```python
from build123d import *

# Parameters (mm, degrees)
BOSS_EXTRUDE1_DEPTH            = 6
CBORE_FOR_M6_SHCS1_D           = 7
CBORE_FOR_M6_SHCS1_CBORE_D     = 10.5
CBORE_FOR_M6_SHCS1_CBORE_DEPTH = 5
FILLET1_R                      = 1


with BuildPart() as part:
    # Sketch1 → Boss-Extrude1 (new, symmetric)
    with BuildSketch(Plane.XY):
        Polygon((-15, 13), (-15, 3), (-4, 3), (-4, 0), (4, 0), (4, 3), (15, 3), (15, 13), align=None)
    extrude(amount=BOSS_EXTRUDE1_DEPTH, both=True)

    # CBORE for M6 SHCS1 (through all)
    with Locations(Plane(origin=(0, 13, 0), x_dir=(1, 0, 0), z_dir=(0, 1, 0))):
        with Locations((0, 0)):
            CounterBoreHole(CBORE_FOR_M6_SHCS1_D / 2, CBORE_FOR_M6_SHCS1_CBORE_D / 2, CBORE_FOR_M6_SHCS1_CBORE_DEPTH)

    # Fillet1
    # the kernel refuses this fillet: 1 mm, written as the material it takes off along each edge
    with BuildSketch(Plane(origin=(-3, 1, 5), x_dir=(-1, 0, 0), z_dir=(0, 0, 1))) as fillet1_piece_1_section:
        Polygon((0, 0), (FILLET1_R, 0), (FILLET1_R, FILLET1_R), (0, FILLET1_R), align=None)
    fillet1_piece_1 = extrude(amount=FILLET1_R, mode=Mode.PRIVATE)
    fillet1_piece_1 = fillet1_piece_1 - Plane(origin=(-3, 1, 5), x_dir=(0.7071067811865475, 0.7071067811865475, 0), z_dir=(0, 0, 1)) * Sphere(FILLET1_R, mode=Mode.PRIVATE)
    add(fillet1_piece_1, mode=Mode.SUBTRACT)
    with BuildSketch(Plane(origin=(3, 1, -5), x_dir=(0, -1, 0), z_dir=(0, 0, -1))) as fillet1_piece_2_section:
        Polygon((0, 0), (FILLET1_R, 0), (FILLET1_R, -FILLET1_R), (0, -FILLET1_R), align=None)
    fillet1_piece_2 = extrude(amount=FILLET1_R, mode=Mode.PRIVATE)
    fillet1_piece_2 = fillet1_piece_2 - Plane(origin=(3, 1, -5), x_dir=(-0.7071067811865475, 0.7071067811865475, 0), z_dir=(0, 0, -1)) * Sphere(FILLET1_R, mode=Mode.PRIVATE)
    add(fillet1_piece_2, mode=Mode.SUBTRACT)
    with BuildSketch(Plane(origin=(3, 1, 5), x_dir=(0, -1, 0), z_dir=(0, 0, 1))) as fillet1_piece_3_section:
        Polygon((0, 0), (FILLET1_R, 0), (FILLET1_R, FILLET1_R), (0, FILLET1_R), align=None)
    fillet1_piece_3 = extrude(amount=FILLET1_R, mode=Mode.PRIVATE)
    fillet1_piece_3 = fillet1_piece_3 - Plane(origin=(3, 1, 5), x_dir=(-0.7071067811865475, 0.7071067811865475, 0), z_dir=(0, 0, 1)) * Sphere(FILLET1_R, mode=Mode.PRIVATE)
    add(fillet1_piece_3, mode=Mode.SUBTRACT)
    with BuildSketch(Plane(origin=(-3, 1, -5), x_dir=(-1, 0, 0), z_dir=(0, 0, -1))) as fillet1_piece_4_section:
        Polygon((0, 0), (FILLET1_R, 0), (FILLET1_R, -FILLET1_R), (0, -FILLET1_R), align=None)
    fillet1_piece_4 = extrude(amount=FILLET1_R, mode=Mode.PRIVATE)
    fillet1_piece_4 = fillet1_piece_4 - Plane(origin=(-3, 1, -5), x_dir=(0.7071067811865475, 0.7071067811865475, 0), z_dir=(0, 0, -1)) * Sphere(FILLET1_R, mode=Mode.PRIVATE)
    add(fillet1_piece_4, mode=Mode.SUBTRACT)
    with BuildSketch(Plane(origin=(-15, 15.5, -6), x_dir=(0, 0, 1), z_dir=(0, -1, 0)), Plane(origin=(15, 0.5, 6), x_dir=(-1, 0, 0), z_dir=(0, 1, 0))) as fillet1_piece_5:
        with BuildLine():
            CenterArc((FILLET1_R, -FILLET1_R), FILLET1_R, 90, 90)
            Line((0, -FILLET1_R), (0, 0))
            Line((0, 0), (FILLET1_R, 0))
        make_face()
    extrude(amount=15, mode=Mode.SUBTRACT)
    with BuildSketch(Plane(origin=(-4, 3, 6), x_dir=(1, 0, 0), z_dir=(0, -1, 0)), Plane(origin=(4, 1, 6), x_dir=(-1, 0, 0), z_dir=(0, 1, 0))) as fillet1_piece_6:
        with BuildLine():
            CenterArc((FILLET1_R, -FILLET1_R), FILLET1_R, 90, 90)
            Line((0, -FILLET1_R), (0, 0))
            Line((0, 0), (FILLET1_R, 0))
        make_face()
    extrude(amount=2, mode=Mode.SUBTRACT)
    with BuildSketch(Plane(origin=(4, 0, -5), x_dir=(-1, 0, 0), z_dir=(0, 0, 1)), Plane(origin=(-4, 0, -5), x_dir=(0, 1, 0), z_dir=(0, 0, 1))) as fillet1_piece_7:
        with BuildLine():
            CenterArc((FILLET1_R, -FILLET1_R), FILLET1_R, 90, 90)
            Line((0, -FILLET1_R), (0, 0))
            Line((0, 0), (FILLET1_R, 0))
        make_face()
    extrude(amount=10, mode=Mode.SUBTRACT)
    with BuildSketch(Plane(origin=(-3, 0, 6), x_dir=(0, 1, 0), z_dir=(1, 0, 0))) as fillet1_piece_8:
        with BuildLine():
            CenterArc((FILLET1_R, -FILLET1_R), FILLET1_R, 90, 90)
            Line((0, -FILLET1_R), (0, 0))
            Line((0, 0), (FILLET1_R, 0))
        make_face()
    extrude(amount=6, mode=Mode.SUBTRACT)
    with BuildSketch(Plane(origin=(-15, 15.5, 6), x_dir=(0, 0, -1), z_dir=(0, -1, 0)), Plane(origin=(15, 0.5, -6), x_dir=(-1, 0, 0), z_dir=(0, 1, 0))) as fillet1_piece_9:
        with BuildLine():
            CenterArc((FILLET1_R, FILLET1_R), FILLET1_R, 180, 90)
            Line((0, FILLET1_R), (0, 0))
            Line((0, 0), (FILLET1_R, 0))
        make_face()
    extrude(amount=15, mode=Mode.SUBTRACT)
    with BuildSketch(Plane(origin=(4, 1, -6), x_dir=(-1, 0, 0), z_dir=(0, 1, 0)), Plane(origin=(-4, 3, -6), x_dir=(1, 0, 0), z_dir=(0, -1, 0))) as fillet1_piece_10:
        with BuildLine():
            CenterArc((FILLET1_R, FILLET1_R), FILLET1_R, 180, 90)
            Line((0, FILLET1_R), (0, 0))
            Line((0, 0), (FILLET1_R, 0))
        make_face()
    extrude(amount=2, mode=Mode.SUBTRACT)
    with BuildSketch(Plane(origin=(-3, 0, -6), x_dir=(0, 1, 0), z_dir=(1, 0, 0))) as fillet1_piece_11:
        with BuildLine():
            CenterArc((FILLET1_R, FILLET1_R), FILLET1_R, 180, 90)
            Line((0, FILLET1_R), (0, 0))
            Line((0, 0), (FILLET1_R, 0))
        make_face()
    extrude(amount=6, mode=Mode.SUBTRACT)


solid = part.part
```
Input: part model. Units: mm. Frame: model coordinates. A direction names the side the tool comes from. Round coordinates to 2 decimals unless told otherwise and drop trailing zeros. Loops run counter-clockwise (first coordinate to the right, second up) from the corner with the lowest first, then second, coordinate; pieces in that order, holes last. Notation, with made-up numbers: M 84,-32.75 L 129,-32.75 A20 ccw 129,-20.75 Z; hole C 15,45.5 d10. An arc over 180 degrees is marked long. Answer in a Markdown table with one row per item. Add a question column.
1. Section A-A (y = 7.25). Output: boundary loops of the cut face in (x, z).
2. Contact query for flat-ended pins moving along their axis: pin 1 (6 mm diameter, centred on x = -8, z = -2.5, fed in from -Y); pin 2 (0.6 mm diameter, centred on y = 2.5, z = 0.5, fed in from +X). Output: stop coordinate, or through.
3. Section C-C (z = -0.75). Output: boundary loops of the cut face in (x, y), and give its area (3 significant figures).
4. Section B-B (x = 0). Output: boundary loops of the cut face in (y, z), and give its area (3 significant figures).
5. Ray query, probe 1 along Z at (x, y) = (0, 9.35); probe 2 along Z at (x, y) = (0, 3.25); probe 3 along Y at (x, z) = (11, 3.5). Return the intervals inside material, ascending.
6. Mould query, pull axis Z, two halves, no side actions, for faces 4 (the face through (-3.233, 3.944, 1.341)), 5 (the face through (15, 8, 0)), 6 (the face through (0, 8, -4)), 7 (the face through (-14.715, 8.07, -5.699)). Classes: released by +Z, released by -Z, zero draft, split by the parting line, or undercut.
7. Set-up query: faces 1 (the face through (3.715, 1.986, -5.699)), 2 (the face through (-3.699, 2.014, 5.715)), 3 (the face through (3.699, 1.986, 5.715)). Return all of +Z, -Z, +X, -X, +Y, -Y with unobstructed straight access to the full face (end or side cutting, diameter ignored); none if empty.
8. Section D-D (z = 0.5). Output: boundary loops of the cut face in (x, y), and give its area (3 significant figures).
Values follow:
| question | item | result |
|---|---|---|
| 1 | outline | M -15,-5 A1 ccw -14,-6 L 14,-6 A1 ccw 15,-5 L 15,5 A1 ccw 14,6 L -14,6 A1 ccw -15,5 Z; hole C 0,0 d7 |
| 2 | pin 1 | y = 3 |
| 2 | pin 2 | x = 4 |
| 3 | outline | M -15,3 L -4,3 L -4,1 A1 ccw -3.42,0.09 L -3.42,8 L -5.2,8 L -5.2,13 L -15,13 Z; M 3.42,0.09 A1 ccw 4,1 L 4,3 L 15,3 L 15,13 L 5.2,13 L 5.2,8 L 3.42,8 Z |
| 3 | area | 217 mm^2 |
| 4 | outline | M 0,-5 A1 ccw 1,-6 L 13,-6 L 13,-5.25 L 8,-5.25 L 8,-3.5 L 0,-3.5 Z; M 0,3.5 L 8,3.5 L 8,5.25 L 13,5.25 L 13,6 L 1,6 A1 ccw 0,5 Z |
| 4 | area | 47.1 mm^2 |
| 5 | probe 1 | -6 to -5.25, 5.25 to 6 |
| 5 | probe 2 | -6 to -3.5, 3.5 to 6 |
| 5 | probe 3 | 3 to 13 |
| 6 | face 4 | undercut |
| 6 | face 5 | zero draft |
| 6 | face 6 | undercut |
| 6 | face 7 | released by -Z |
| 7 | face 1 | -Z, +X, -Y |
| 7 | face 2 | +Z, -X, -Y |
| 7 | face 3 | +Z, +X, -Y |
| 8 | outline | M -15,3 L -4,3 L -4,1 A1 ccw -3.46,0.11 L -3.46,8 L -5.23,8 L -5.23,13 L -15,13 Z; M 3.46,0.11 A1 ccw 4,1 L 4,3 L 15,3 L 15,13 L 5.23,13 L 5.23,8 L 3.46,8 Z |
| 8 | area | 216 mm^2 |
